Work out the finished part from the listing and answer in its coordinate system (mm). A direction names the side the tool comes from. Give positions to 0.01 mm unless a question says otherwise; leave off trailing zeros. Loops run counter-clockwise (first coordinate to the right, second up) from the corner with the lowest first, then second, coordinate; pieces in that order, holes last. Notation, with made-up numbers: (19, 28) -> (50, 28) arc R22 cw to (50, 56) -> close; hole circle Ø8 at (18.25, -15). An arc over 180 degrees is marked (long way). Answer as CSV lines item,"result". Start each with the question number.
1. Find section B-B, the plane y = -24.5. Give the vertices of the cut face in (x, z), and give its area (3 significant figures).
2. Find section A-A, the plane x = 0. Give the vertices of the cut face in (y, z) (3 decimals).
3. Find the intervals of material crossed by line 1 along Y through (x, z) = (0, 0.65) (3 decimals); line 2 along X through (y, z) = (-24, 8); line 3 along Y through (x, z) = (-3, 5), in increasing order.
4. A tool of negligible diameter and unlimited length cuts with its end or side. For faces 4 (the face through (1, -32.5, 4)), 5 (the face through (8.5, -24, 6)), 6 (the face through (0.044, 19.425, 1.232)), from which of +Z, -Z, +X, -X, +Y, -Y can it reach the whole face along a straight path? Write none if from no direction.
5. Find section C-C, the plane z = 6.5. Give the vertices of the cut face in (x, y), and give its area (3 significant figures).
6. Determine the mould class of faces 1 (the face through (-60, 0, 4)), 2 (the face through (-1, 32.5, 4)), 3 (the face through (0, -30.3, 6)) for opening direction Y: +Y half, -Y half, draft (parallel to the pull), parting line (faces both ways), or undercut.
7. Flat-ended cylindrical pins translate along their axes: pin 1 Ø9.5 at (x, y) = (-1.5, -25) entering from +Z; pin 2 Ø6.5 at (x, y) = (0, -24.5) entering from +Z. Find the tip coordinate at first contact, or state that the pin passes through.
Autodesk Inventor part; units mm, degrees
ref_plane "YZ Plane" through (0, 0, 0) normal (1, 0, 0) x (0, 1, 0)
ref_plane "XZ Plane" through (0, 0, 0) normal (0, 1, 0) x (-1, 0, 0)
ref_plane "XY Plane" through (0, 0, 0) normal (0, 0, 1) x (1, 0, 0)
sketch "Schizzo1" plane through (0, 0, 0) normal (0, 0, 1) x (1, 0, 0)
  line L0 (-60, 32.5) -> (60, 32.5)
  line L1 (60, 32.5) -> (60, -32.5)
  line L2 (60, -32.5) -> (-60, -32.5)
  line L3 (-60, -32.5) -> (-60, 32.5)
  line L4 (-60, 32.5) -> (60, -32.5) construction
  line L5 (60, 32.5) -> (-60, -32.5) construction
  line L6 (-8.5, -18.7) -> (8.5, -18.7)
  line L7 (8.5, -18.7) -> (8.5, -30.3)
  line L8 (8.5, -30.3) -> (-8.5, -30.3)
  line L9 (-8.5, -30.3) -> (-8.5, -18.7)
  line L10 (-8.5, -18.7) -> (8.5, -30.3) construction
  line L11 (8.5, -18.7) -> (-8.5, -30.3) construction
  line L12 (-12, 12) -> (12, -12) construction
  line L13 (12, 12) -> (-12, -12) construction
  line L14 (-8.95, 29.85) -> (8.95, 29.85)
  line L15 (8.95, 29.85) -> (8.95, 17)
  line L16 (8.95, 17) -> (-8.95, 17)
  line L17 (-8.95, 17) -> (-8.95, 29.85)
  line L18 (-8.95, 29.85) -> (8.95, 17) construction
  line L19 (8.95, 29.85) -> (-8.95, 17) construction
  circle A0 centre (0, -24.5) radius 4.1
  line L20 (0, 25.425) -> (0, 21.425) construction
  line L21 (-2, 25.425) -> (-2, 21.425)
  line L22 (2, 21.425) -> (2, 25.425)
  arc A1 (2, 25.425) -> (-2, 25.425) centre (0, 25.425) ccw
  arc A2 (-2, 21.425) -> (2, 21.425) centre (0, 21.425) ccw
  point P0 (0, 0)
  point P1 (0, 0)
  point P2 (0, 23.425)
  dimension "d0" = 120
  dimension "d1" = 65
  dimension "d2" = 17
  dimension "d3" = 11.6
  dimension "d4" = 24
  dimension "d5" = 24
  dimension "d6" = 17.9
  dimension "d7" = 12.85
  dimension "d8" = 8.2
  dimension "d9" = 2
  dimension "d10" = 4
extrude "Estrusione1" add sketch "Schizzo1" along normal blind 9 contours L0 L1 L2 L3
sketch "Schizzo2" plane through (0, 0, 0) normal (0, 0, -1) x (-1, 0, 0)
  line L0 (-60, 32.5) -> (60, 32.5)
  line L1 (60, 32.5) -> (60, -32.5)
  line L2 (60, -32.5) -> (-60, -32.5)
  line L3 (-60, -32.5) -> (-60, 32.5)
  line L4 (-60, 32.5) -> (60, -32.5) construction
  line L5 (60, 32.5) -> (-60, -32.5) construction
  line L6 (-8.95, 17) -> (-8.95, 29.85)
  line L7 (-12, 12) -> (12, -12) construction
  line L8 (12, 12) -> (-12, -12) construction
  line L9 (8.95, 17) -> (-8.95, 17)
  line L10 (-8.95, 29.85) -> (8.95, 29.85)
  line L11 (8.95, 29.85) -> (-8.95, 17) construction
  line L12 (8.95, 29.85) -> (8.95, 17)
  line L13 (-8.95, 29.85) -> (8.95, 17) construction
  line L14 (-8.5, -18.7) -> (8.5, -18.7)
  line L15 (8.5, -18.7) -> (8.5, -30.3)
  line L16 (8.5, -30.3) -> (-8.5, -30.3)
  line L17 (-8.5, -30.3) -> (-8.5, -18.7)
  line L18 (-8.5, -18.7) -> (8.5, -30.3) construction
  line L19 (8.5, -18.7) -> (-8.5, -30.3) construction
  circle A0 centre (0, -24.5) radius 4.1
  line L20 (0, 25.425) -> (0, 21.425) construction
  line L21 (-2, 25.425) -> (-2, 21.425)
  line L22 (2, 21.425) -> (2, 25.425)
  arc A1 (2, 25.425) -> (-2, 25.425) centre (0, 25.425) ccw
  arc A2 (-2, 21.425) -> (2, 21.425) centre (0, 21.425) ccw
  point P0 (0, 0)
  point P1 (0, 0)
  point P2 (0, 0)
  point P3 (0, 23.425)
  dimension "d13" = 120
  dimension "d14" = 65
  dimension "d15" = 17
  dimension "d16" = 11.6
  dimension "d17" = 24
  dimension "d18" = 24
  dimension "d19" = 17.9
  dimension "d20" = 12.85
  dimension "d21" = 8.2
  dimension "d22" = 2
  dimension "d23" = 4
extrude "Estrusione2" add sketch "Schizzo2" against normal blind 2.5 contours L6 L10 L12 L9 | L14 L15 L16 L17
Resolved:
1,outline,"(-60, 0) -> (-4.1, 0) -> (-4.1, 2.5) -> (-8.5, 2.5) -> (-8.5, 9) -> (-60, 9) -> close; (4.1, 0) -> (60, 0) -> (60, 9) -> (8.5, 9) -> (8.5, 2.5) -> (4.1, 2.5) -> close"
1,area,"949 mm^2"
2,outline,"(-32.5, 0) -> (-28.6, 0) -> (-28.6, 2.5) -> (-30.3, 2.5) -> (-30.3, 9) -> (-32.5, 9) -> close; (-20.4, 0) -> (19.425, 0) -> (19.425, 2.5) -> (17, 2.5) -> (17, 9) -> (-18.7, 9) -> (-18.7, 2.5) -> (-20.4, 2.5) -> close; (27.425, 0) -> (32.5, 0) -> (32.5, 9) -> (29.85, 9) -> (29.85, 2.5) -> (27.425, 2.5) -> close"
3,line 1,"y = -32.5 to -28.6, -20.4 to 19.425, 27.425 to 32.5"
3,line 2,"x = -60 to -8.5, 8.5 to 60"
3,line 3,"y = -32.5 to -30.3, -18.7 to 17, 29.85 to 32.5"
4,face 4,"+Z, -Z, +X, -X, -Y"
4,face 5,"+Z"
4,face 6,"+Z, -Z"
5,outline,"(-60, -32.5) -> (60, -32.5) -> (60, 32.5) -> (-60, 32.5) -> close; hole (-8.95, 17) -> (8.95, 17) -> (8.95, 29.85) -> (-8.95, 29.85) -> close; hole (-8.5, -30.3) -> (8.5, -30.3) -> (8.5, -18.7) -> (-8.5, -18.7) -> close"
5,area,"7,370 mm^2"
6,face 1,"draft"
6,face 2,"+Y half"
6,face 3,"undercut"
7,pin 1,"stops at z = 2.5"
7,pin 2,"passes through"
